Solid Edge part; units mm, degrees
sketch "Sketch1" plane through (0, 0, 0) normal (0, 0, 1) x (1, 0, 0)
  line L0 (21, -21) -> (21, 21)
  line L1 (21, 21) -> (-21, 21)
  line L2 (-21, 21) -> (-21, -21)
  line L3 (-21, -21) -> (21, -21)
extrude "Protrusion1" add sketch "Sketch1" along normal mid plane 47
sketch "Sketch2" plane through (0, 0, 0) normal (0, 0, 1) x (1, 0, 0)
  line L0 (20.5, -20.5) -> (20.5, 20.5)
  line L1 (20.5, 20.5) -> (-20.5, 20.5)
  line L2 (-20.5, 20.5) -> (-20.5, -20.5)
  line L3 (-20.5, -20.5) -> (20.5, -20.5)
extrude "VaciadoExtruido_1" cut sketch "Sketch2" along normal mid plane 31 flip side to cut
chamfer "Chaflán_1" distance 8 angle 45 4 edges at (20.5, -20.5, 0) (20.5, 20.5, 0) (-20.5, -20.5, 0) (-20.5, 20.5, 0)
chamfer "Chaflán_2" distance 4 angle 45 8 edges at (21, -21, 19.5) (21, 21, 19.5) (21, 21, -19.5) (21, -21, -19.5) (-21, -21, -19.5) (-21, -21, 19.5) (-21, 21, 19.5) (-21, 21, -19.5)
fillet "Redondeo_1" radius 2 8 edges at (-20.5, 12.5, 0) (-12.5, 20.5, 0) (12.5, 20.5, 0) (20.5, 12.5, 0) (20.5, -12.5, 0) (12.5, -20.5, 0) (-12.5, -20.5, 0) (-20.5, -12.5, 0)
fillet "Redondeo_2" radius 1 16 edges at (-21, -17, 19.5) (-17, -21, 19.5) (-21, 17, 19.5) (-17, 21, 19.5) (17, -21, 19.5) (21, -17, 19.5) (21, 17, 19.5) (17, 21, 19.5) (21, 17, -19.5) (21, -17, -19.5) (17, -21, -19.5) (-17, -21, -19.5) (-21, -17, -19.5) (-21, 17, -19.5) (-17, 21, -19.5) (17, 21, -19.5)
sketch "Sketch3" plane through (0, 0, 23.5) normal (0, 0, 1) x (0, 1, 0)
  circle A0 centre (0, 0) radius 11
extrude "ProtrusiónExtruida_3" add sketch "Sketch3" along normal blind 1.5
sketch "Sketch4" plane through (0, 0, 25) normal (0, 0, 1) x (0, 1, 0)
  line L0 (-1.5, 2) -> (1.5, 2)
  arc A0 (1.5, 2) -> (-1.5, 2) centre (0, 0) cw
extrude "ProtrusiónExtruida_4" add sketch "Sketch4" along normal blind 22
hole "Agujero_1" at (-15.5, -15.5, 23.5) direction (0, 0, -1) diameter 3 depth 5
hole "Hole1" at (15.5, -15.5, 23.5) direction (0, 0, -1) diameter 3 depth 5
hole "Hole2" at (15.5, 15.5, 23.5) direction (0, 0, -1) diameter 3 depth 5
hole "Hole3" at (-15.5, 15.5, 23.5) direction (0, 0, -1) diameter 3 depth 5
chamfer "Chaflán_3" distance 0.5 angle 45 4 edges at (-15.5, -14, 23.5) (-15.5, 17, 23.5) (15.5, 17, 23.5) (15.5, -14, 23.5)
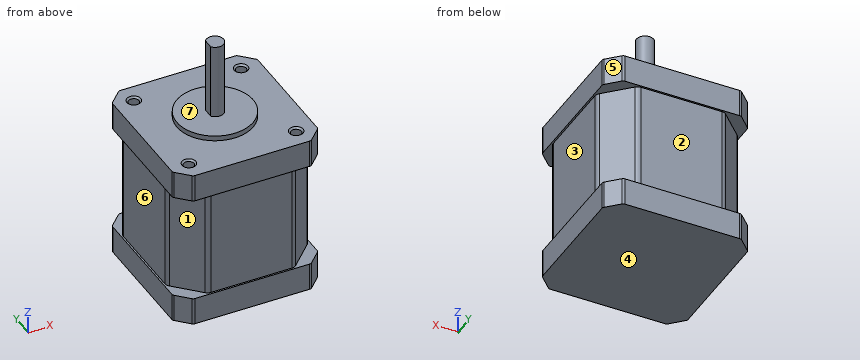
CAD build for the part. Positions are in the model's coordinates, mm. Face numbers are marked on the shaded views. A direction names the side the tool comes from. Round coordinates to 2 decimals unless told otherwise and drop trailing zeros. Write each loop counter-clockwise with the first axis right and the second up, starting at its lowest first coordinate (ties: lowest second). Pieces come first, ordered by that corner, then holes. Notation, with made-up numbers: (76, 50) -> (120, 50) arc R37 ccw to (120, 87) -> close; hole circle Ø2 at (26.25, 33.5). An arc over 180 degrees is marked (long way). Answer in a Markdown table with one row per item. Add a question column.
Item 1: Drill centre lines: line 1 (Y direction, x = -15.5, z = 19.95); line 2 (Z direction, x = -18.5, y = -15). Where is each one in solid material? Low to high. Write a range as from..to.
Item 2: Mould opens along Z. For the marked faces 4, 5, 6 and 7 say: pulls with the +Z half, pulls with the -Z half, needs draft (parallel to the pull), parting line crosses it, or undercut.
Item 3: Which spindle directions (+Z, -Z, +X, -X, +Y, -Y) get a long thin tool onto all of the face, cutting with end or side? Do the marked faces 1, 2 and 3. Say none if no direction does.
Item 4: Saw through at C-C, the plane x = -15.5. Write the cut outline in (y, z), then the cut area to 3 significant figures.
Item 5: Saw through at D-D, the plane z = -3. Write the cut outline in (x, y), then the cut area to 3 significant figures.
Item 6: Drop flat-ended pins along their axis: pin 1 Ø1 at (x, z) = (-10.5, -11.5) entering from -Y; pin 2 Ø2.5 at (x, y) = (-15, -15) entering from +Z; pin 3 Ø21 at (x, y) = (6, -8.5) entering from +Z; pin 4 Ø18.5 at (y, z) = (4, 5.5) entering from -X. Give the stop position or say it passes through.
Item 7: Saw through at B-B, the plane z = 17. Write the cut outline in (x, y), then the cut area to 3 significant figures.
Item 8: Saw through at A-A, the plane y = 0. Write the cut outline in (x, z).
Findings below:
| question | item | result |
|---|---|---|
| 1 | line 1 | y = -21..-17, -14..14, 17..21 |
| 1 | line 2 | z = -23.5..-15.5, 15.5..23.5 |
| 2 | face 4 | pulls with the -Z half |
| 2 | face 5 | needs draft |
| 2 | face 6 | undercut |
| 2 | face 7 | pulls with the +Z half |
| 3 | face 1 | -X, -Y |
| 3 | face 2 | +X, -X, +Y |
| 3 | face 3 | +X, +Y, -Y |
| 4 | outline | (-21, -23.5) -> (21, -23.5) -> (21, -15.5) -> (17.5, -15.5) -> (17.5, 15.5) -> (21, 15.5) -> (21, 23.5) -> (17.5, 23.5) -> (17, 23) -> (17, 18.5) -> (14, 18.5) -> (14, 23) -> (13.5, 23.5) -> (-13.5, 23.5) -> (-14, 23) -> (-14, 18.5) -> (-17, 18.5) -> (-17, 23) -> (-17.5, 23.5) -> (-21, 23.5) -> (-21, 15.5) -> (-17.5, 15.5) -> (-17.5, -15.5) -> (-21, -15.5) -> close |
| 4 | area | 1,730 mm^2 |
| 5 | outline | (-20.5, -11.67) arc R2 ccw to (-19.91, -13.09) -> (-13.09, -19.91) arc R2 ccw to (-11.67, -20.5) -> (11.67, -20.5) arc R2 ccw to (13.09, -19.91) -> (19.91, -13.09) arc R2 ccw to (20.5, -11.67) -> (20.5, 11.67) arc R2 ccw to (19.91, 13.09) -> (13.09, 19.91) arc R2 ccw to (11.67, 20.5) -> (-11.67, 20.5) arc R2 ccw to (-13.09, 19.91) -> (-19.91, 13.09) arc R2 ccw to (-20.5, 11.67) -> close |
| 5 | area | 1,550 mm^2 |
| 6 | pin 1 | stops at y = -20.5 |
| 6 | pin 2 | stops at z = 23.46 |
| 6 | pin 3 | stops at z = 47 |
| 6 | pin 4 | stops at x = -20.5 |
| 7 | outline | (-21, -16.59) arc R1 ccw to (-20.71, -17.29) -> (-17.29, -20.71) arc R1 ccw to (-16.59, -21) -> (16.59, -21) arc R1 ccw to (17.29, -20.71) -> (20.71, -17.29) arc R1 ccw to (21, -16.59) -> (21, 16.59) arc R1 ccw to (20.71, 17.29) -> (17.29, 20.71) arc R1 ccw to (16.59, 21) -> (-16.59, 21) arc R1 ccw to (-17.29, 20.71) -> (-20.71, 17.29) arc R1 ccw to (-21, 16.59) -> close |
| 7 | area | 1,730 mm^2 |
| 8 | outline | (-21, -23.5) -> (21, -23.5) -> (21, -15.5) -> (20.5, -15.5) -> (20.5, 15.5) -> (21, 15.5) -> (21, 23.5) -> (11, 23.5) -> (11, 25) -> (2.5, 25) -> (2.5, 47) -> (-2, 47) -> (-2, 25) -> (-11, 25) -> (-11, 23.5) -> (-21, 23.5) -> (-21, 15.5) -> (-20.5, 15.5) -> (-20.5, -15.5) -> (-21, -15.5) -> close |
